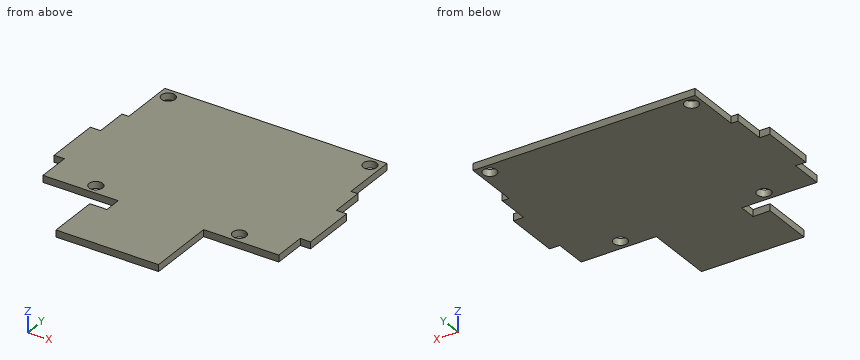
```python
from build123d import *

# Parameters (mm, degrees)
F0_R     = 2
F1_DEPTH = 2


with BuildPart() as f1:
    # F0 (on Top) → F1 (new body)
    with BuildSketch(Plane.XY):
        Polygon((32.5, 9.5), (32.5, 25.5), (-32.5, 25.5), (-32.5, 9.5), (-32.5, -25.5), (-12.5, -25.5), (12.5, -25.5), (32.5, -25.5), align=None)
        with Locations((-21, -22.5)):
            Circle(F0_R, mode=Mode.SUBTRACT)
        with Locations((21, -22.5)):
            Circle(F0_R, mode=Mode.SUBTRACT)
        with Locations((-29.5, 22.5)):
            Circle(F0_R, mode=Mode.SUBTRACT)
        with Locations((29.5, 22.5)):
            Circle(F0_R, mode=Mode.SUBTRACT)
        Polygon((34.5, 9.5), (32.5, 9.5), (32.5, -25.5), (34.5, -25.5), (34.5, -16), (37.5, -16), (37.5, 0), (34.5, 0), align=None)
        Polygon((-32.5, -25.5), (-32.5, 9.5), (-34.5, 9.5), (-34.5, 0), (-37.5, 0), (-37.5, -16), (-34.5, -16), (-34.5, -25.5), align=None)
        Polygon((12.5, -45.5), (12.5, -25.5), (-12.5, -25.5), (-12.5, -30.5), (-17.5, -30.5), (-17.5, -45.5), align=None)
    extrude(amount=F1_DEPTH)


solid = f1.part
```
CAD build for the part. Positions are in the model's coordinates, mm. Round coordinates to 2 decimals unless told otherwise and drop trailing zeros. Order: outer loops, then holes, each group sorted by start corner. A loop starts at its lowest first (then second) coordinate and runs counter-clockwise, first axis right, second up. Notation, with made-up numbers: (12, 88) -> (54, 88) arc R31 ccw to (54, 119) -> close; hole circle Ø4 at (-14.5, 65.25). An arc over 180 degrees is marked (long way). One line per question, with ' | ' between items.
Q1. Slice it at A-A (y = -22.5). Write the cut outline in (x, z), then the cut area to 3 significant figures.
Completed:
outline: (-34.5, 0) -> (-23, 0) -> (-23, 2) -> (-34.5, 2) -> close; (-19, 0) -> (19, 0) -> (19, 2) -> (-19, 2) -> close; (23, 0) -> (34.5, 0) -> (34.5, 2) -> (23, 2) -> close | area: 122 mm^2
Q2. Slice it at B-B (x = -21). Write the cut outline in (y, z), then the cut area to 3 significant figures.
Completed:
outline: (-25.5, 0) -> (-24.5, 0) -> (-24.5, 2) -> (-25.5, 2) -> close; (-20.5, 0) -> (25.5, 0) -> (25.5, 2) -> (-20.5, 2) -> close | area: 94.0 mm^2
Q3. Slice it at C-C (z = 0.35). Write the cut outline in (x, y), then the cut area to 3 significant figures.
Completed:
outline: (-37.5, -16) -> (-34.5, -16) -> (-34.5, -25.5) -> (-12.5, -25.5) -> (-12.5, -30.5) -> (-17.5, -30.5) -> (-17.5, -45.5) -> (12.5, -45.5) -> (12.5, -25.5) -> (34.5, -25.5) -> (34.5, -16) -> (37.5, -16) -> (37.5, 0) -> (34.5, 0) -> (34.5, 9.5) -> (32.5, 9.5) -> (32.5, 25.5) -> (-32.5, 25.5) -> (-32.5, 9.5) -> (-34.5, 9.5) -> (-34.5, 0) -> (-37.5, 0) -> close; hole circle Ø4 at (-29.5, 22.5); hole circle Ø4 at (-21, -22.5); hole circle Ø4 at (21, -22.5); hole circle Ø4 at (29.5, 22.5) | area: 4,080 mm^2
Q4. Probe probe 1 along Y at (x, z) = (29.5, 0.7); probe 2 along Y at (x, z) = (-21, 0.95); probe 3 along Y at (x, z) = (-26, 1.15). List the from-to ranges inside material, lowest first.
Completed:
probe 1: y = -25.5 to 20.5, 24.5 to 25.5 | probe 2: y = -25.5 to -24.5, -20.5 to 25.5 | probe 3: y = -25.5 to 25.5
Q5. Slice it at D-D (y = 22.5). Write the cut outline in (x, z), then the cut area to 3 significant figures.
Completed:
outline: (-32.5, 0) -> (-31.5, 0) -> (-31.5, 2) -> (-32.5, 2) -> close; (-27.5, 0) -> (27.5, 0) -> (27.5, 2) -> (-27.5, 2) -> close; (31.5, 0) -> (32.5, 0) -> (32.5, 2) -> (31.5, 2) -> close | area: 114 mm^2
Q6. Drop flat-ended pins along their axis: pin 1 (1 mm diameter, centred on y = 2.5, z = 1.5, fed in from +X); pin 2 (1 mm diameter, centred on x = 34, z = 1, fed in from +Y); pin 3 (1 mm diameter, centred on y = -36.5, z = 1.5, fed in from +X); pin 4 (2.5 mm diameter, centred on x = 29.5, y = 22.5, fed in from +Z). Give the stop position or say it passes through.
Completed:
pin 1: stops at x = 34.5 | pin 2: stops at y = 9.5 | pin 3: stops at x = 12.5 | pin 4: passes through
